```python
from build123d import *

# Parameters (mm, degrees)
F1_DEPTH       = 14
F3_D           = 4.4
F3_CBORE_D     = 8.25
F3_CBORE_DEPTH = 4
F4_T1_DEPTH    = 14
F4_T3_DEPTH    = 19
F6_D           = 5.5


# Not quite as in the source:
# - a fillet or chamfer that OpenCascade refuses, or shapes differently, is made with other operations: its cross-section is extruded or revolved along the edge and cut away or added


with BuildPart() as f1:
    # F0 (on Front) → F1 (new body)
    with BuildSketch(Plane.XZ):
        with BuildLine():
            Line((-21, 6), (-21, 0))
            Line((-21, 0), (21, 0))
            Line((21, 0), (21, 6))
            Line((21, 6), (9, 6))
            Line((9, 6), (9, 32.8))
            Line((9, 32.8), (1, 32.8))
            Line((1, 32.8), (1, 23.8729833462))
            ThreePointArc((1, 23.8729833462), (3.1622776602, 22.4494897428), (4, 20))
            ThreePointArc((4, 20), (-2.4494897428, 16.8377223398), (-1, 23.8729833462))
            Line((-1, 23.8729833462), (-1, 32.8))
            Line((-1, 32.8), (-9, 32.8))
            Line((-9, 32.8), (-9, 6))
            Line((-9, 6), (-21, 6))
        make_face()
    extrude(amount=F1_DEPTH)

    # F3 (through all)
    with Locations(Plane.YZ.offset(9)):
        with Locations((-7, 28.3364916731)):
            CounterBoreHole(F3_D / 2, F3_CBORE_D / 2, F3_CBORE_DEPTH)

    # F4: fillet of radius 1 on 6 edges, made by hand

    # F4_s2 → F4_t1 (join)
    with BuildSketch(Plane.XZ):
        with BuildLine():
            ThreePointArc((10, 6), (9.2928932188, 6.2928932188), (9, 7))
            Line((9, 7), (9, 6))
            Line((9, 6), (10, 6))
        make_face()
        with BuildLine():
            ThreePointArc((-9, 7), (-9.2928932188, 6.2928932188), (-10, 6))
            Line((-10, 6), (-9, 6))
            Line((-9, 6), (-9, 7))
        make_face()
    extrude(amount=F4_T1_DEPTH)

    # F4_s4 → F4_t3 (cut)
    with BuildSketch(Plane.XZ.offset(-2.5)):
        with BuildLine():
            ThreePointArc((-20, 6), (-20.7071067812, 5.7071067812), (-21, 5))
            Line((-21, 5), (-21, 6))
            Line((-21, 6), (-20, 6))
        make_face()
        with BuildLine():
            ThreePointArc((21, 5), (20.7071067812, 5.7071067812), (20, 6))
            Line((20, 6), (21, 6))
            Line((21, 6), (21, 5))
        make_face()
        with BuildLine():
            ThreePointArc((-8, 32.8), (-8.7071067812, 32.5071067812), (-9, 31.8))
            Line((-9, 31.8), (-9, 32.8))
            Line((-9, 32.8), (-8, 32.8))
        make_face()
        with BuildLine():
            ThreePointArc((9, 31.8), (8.7071067812, 32.5071067812), (8, 32.8))
            Line((8, 32.8), (9, 32.8))
            Line((9, 32.8), (9, 31.8))
        make_face()
    extrude(amount=F4_T3_DEPTH, mode=Mode.SUBTRACT)

    # F6 (through all)
    with Locations(Plane.XY.offset(6)):
        with Locations((-16, -6.7585341167), (16, -6.7585341167)):
            Hole(F6_D / 2)


solid = f1.part
```
Geometry check sheet. Reference: the model listing, model coordinates, mm. A direction names the side the tool comes from. Round coordinates to 2 decimals unless told otherwise and drop trailing zeros. Order: outer loops, then holes, each group sorted by start corner. A loop starts at its lowest first (then second) coordinate and runs counter-clockwise, first axis right, second up. Notation, with made-up numbers: (19, -3.75) -> (31, -3.75) arc R31 cw to (31, 26.25) -> close; hole circle Ø6 at (-17.5, -2). An arc over 180 degrees is marked (long way). Return JSON: item names as keys, results as strings. Group by question number.
Q1. Section check B-B, the plane z = 17. Record the boundary of the cut face in (x, y), plus the area to 3 significant figures.
Q2. Tool access check on faces 4 (the cylindrical face through (7.028, -5.097, 24.677)), 5 (the flat face through (5, -7, 32.8)), 6 (the flat face through (9, -7, 16)), 7 (the flat face through (-13, -7, 6)), 8 (the flat face through (-1, -8, 26)). Record the directions out of +Z, -Z, +X, -X, +Y, -Y that give a thin tool (end or side, any length) a straight path to the whole face; none if there is none.
Q3. Release check for a two-part mould opening along Z. For faces 1 (the cylindrical face through (-9.285, -6.902, 6.301)), 2 (the flat face through (0, -14, 9)), 3 (the cylindrical face through (-5.056, -8.015, 26.385)) record: released by +Z, released by -Z, zero draft, split by the parting line, or undercut.
Q4. Gauge pin test, flat ends, axial feed: pin 1 (7 mm diameter, centred on y = -7.5, z = 18, fed in from -X); pin 2 (4 mm diameter, centred on y = -10, z = 18.5, fed in from +X); pin 3 (3 mm diameter, centred on x = -11, y = -6.5, fed in from +Z); pin 4 (4.5 mm diameter, centred on x = 16, y = -6.76, fed in from +Z). Record the tip position at first contact, or that the pin passes through.
Q5. Material ranges on probe 1 along X at (y, z) = (-3.5, 26.5); probe 2 along X at (y, z) = (-12.25, 26.5); probe 3 along Y at (x, z) = (-16, 3), recorded low to high. Write a range as from..to.
Q6. Section check A-A, the plane x = 1.5. Record the boundary of the cut face in (y, z), plus the area to 3 significant figures.
Q7. Section check C-C, the plane x = -16. Record the boundary of the cut face in (y, z).
Q8. Section check D-D, the plane y = -2. Record the boundary of the cut face in (x, z).
Numbers:
{
 "1": {"outline": "(-9, -14) -> (-2.65, -14) -> (-2.65, 0) -> (-9, 0) -> close; (2.65, -14) -> (9, -14) -> (9, 0) -> (2.65, 0) -> close", "area": "178 mm^2"},
 "2": {"face 4": "+X", "face 5": "+Z, +X, -X, +Y, -Y", "face 6": "+Z, +X, +Y, -Y", "face 7": "+Z, -X, +Y, -Y", "face 8": "+Z, +Y, -Y"},
 "3": {"face 1": "released by +Z", "face 2": "zero draft", "face 3": "undercut"},
 "4": {"pin 1": "x = -9", "pin 2": "x = 9", "pin 3": "z = 6.13", "pin 4": "through"},
 "5": {"probe 1": "-9..-1, 1..5", "probe 2": "-9..-1, 1..9", "probe 3": "-14..-9.51, -4.01..0"},
 "6": {"outline": "(-14, 0) -> (0, 0) -> (0, 16.29) -> (-14, 16.29) -> close; (-14, 23.71) -> (0, 23.71) -> (0, 32.8) -> (-14, 32.8) -> close; hole circle Ø4.4 at (-7, 28.34)", "area": "340 mm^2"},
 "7": {"outline": "(-14, 0) -> (-9.51, 0) -> (-9.51, 6) -> (-14, 6) -> close; (-4.01, 0) -> (0, 0) -> (0, 6) -> (-4.01, 6) -> close"},
 "8": {"outline": "(-21, 0) -> (21, 0) -> (21, 5) arc R1 ccw to (20, 6) -> (10, 6) arc R1 cw to (9, 7) -> (9, 31.8) arc R1 ccw to (8, 32.8) -> (1, 32.8) -> (1, 23.87) arc R4 cw (long way) to (-1, 23.87) -> (-1, 32.8) -> (-8, 32.8) arc R1 ccw to (-9, 31.8) -> (-9, 7) arc R1 cw to (-10, 6) -> (-20, 6) arc R1 ccw to (-21, 5) -> close"}
}
